For this review, take the finished solid that the model builds, in its own axes (mm). Face numbers are marked on the shaded views. A direction names the side the tool comes from. Coordinates: 2 decimals unless noted, no trailing zeros. Write each loop counter-clockwise with the first axis right and the second up, starting at its lowest first coordinate (ties: lowest second). Pieces come first, ordered by that corner, then holes. Notation, with made-up numbers: (6.25, -12.75) -> (12.25, -12.75) arc R23 cw to (12.25, 4.25) -> close; hole circle Ø2 at (11.25, 50). An arc over 180 degrees is marked (long way). Put each result on its own line as item: value. Start each with the question number.
Item 1: Insertion check: P1, Ø3, axis at x = 47.5, y = 2, coming from the -Z side; P2, Ø1, axis at y = 2.5, z = -10.5, coming from the +X side; P3, Ø3, axis at y = -2.5, z = 2.5, coming from the -X side. Each pin has a flat end and moves straight along its axis. Give the tip position at first contact, or say it passes through.
Item 2: Consider section B-B on y = -1. Give the boundary of the cut face in (x, z), and give its area (3 significant figures).
Item 3: Consider section C-C on x = 14. Give the boundary of the cut face in (y, z) (3 decimals).
Item 4: The part is to be moulded in two halves that separate along X. For the marked faces 3, 4 and 5, say which applies: +X half, -X half, draft (parallel to the pull), parting line (faces both ways), or undercut.
Item 5: To check wall thickness, follow L1, parallel to Z at x = 33.5, y = 1.5; L2, parallel to Z at x = 3, y = -0.5. State the ranges of each line that lie inside material, in increasing order.
Item 6: Consider section A-A on z = 0. Give the boundary of the cut face in (x, y) (3 decimals), and give its area (3 significant figures).
Item 7: Consider section D-D on x = 67.5. Give the boundary of the cut face in (y, z) (3 decimals).
Item 8: For the marked faces 1 and 2, list the 3-axis set-ups (+Z, -Z, +X, -X, +Y, -Y) from which the entire face can be reached by the end or side of a thin tool; tool diameter is ignored.
```python
from build123d import *

# Parameters (mm, degrees)
SKETCH1_R           = 3.2639
BOSS_EXTRUDE1_DEPTH = 3.175
BOSS_EXTRUDE2_START = -6.35
SKETCH3_R           = 2.4892
BOSS_EXTRUDE2_DEPTH = 6.35
FILLET2_R           = 6.35


with BuildPart() as part:
    # Sketch1 → Boss-Extrude1 (new, symmetric)
    with BuildSketch(Plane(origin=(0, 0, 0), x_dir=(1, 0, 0), z_dir=(0, 1, 0))):
        with BuildLine():
            Line((0, 6.35), (50.8, 6.35))
            ThreePointArc((50.8, 6.35), (57.15, 0), (50.8, -6.35))
            Line((50.8, -6.35), (0, -6.35))
            ThreePointArc((0, -6.35), (-6.35, 0), (0, 6.35))
        make_face()
        with Locations(Location((0, 0, 0), (0, 0, 270))):
            Circle(SKETCH1_R, mode=Mode.SUBTRACT)
        with Locations(Location((50.8, 0, 0), (0, 0, 270))):
            Circle(SKETCH1_R, mode=Mode.SUBTRACT)
    extrude(amount=BOSS_EXTRUDE1_DEPTH, both=True)

    # Sketch3 → Boss-Extrude2 (add)
    with BuildSketch(Plane.XZ.offset(3.175).offset(BOSS_EXTRUDE2_START)):
        with BuildLine():
            Line((76.840020478, -2.720263498), (52.97182791, 5.967048142))
            ThreePointArc((52.97182791, 5.967048142), (57.053529232, -1.102665928), (50.8, -6.35))
            Line((50.8, -6.35), (49.680323673, -6.35))
            Line((49.680323673, -6.35), (72.496364658, -14.654359782))
            ThreePointArc((72.496364658, -14.654359782), (80.63524071, -10.859139551), (76.840020478, -2.720263498))
        make_face()
        with Locations(Location((74.668192568, -8.68731164, 0), (0, 0, 270))):
            Circle(SKETCH3_R, mode=Mode.SUBTRACT)
    extrude(amount=BOSS_EXTRUDE2_DEPTH)

    # Fillet2
    fillet2_edges = [part.edges().sort_by_distance(p)[0] for p in [
        (49.680323673, 0, -6.35),
    ]]
    fillet(fillet2_edges, radius=FILLET2_R)


solid = part.part
```
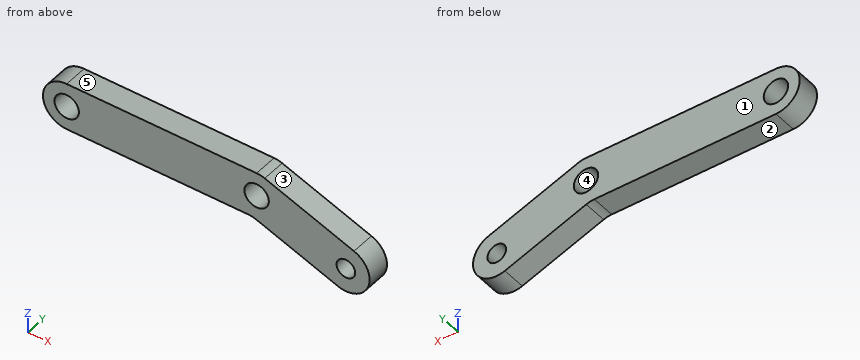
Return value:
1. P1: z = -6.37
1. P2: x = 80.88
1. P3: x = -6.27
2. outline: (0, -6.35) -> (48.56, -6.35) arc R6.35 cw to (50.73, -6.73) -> (72.5, -14.65) arc R6.35 ccw to (76.84, -2.72) -> (52.97, 5.97) arc R6.35 ccw to (50.8, 6.35) -> (0, 6.35) arc R6.35 ccw to start; hole circle Ø6.53 at (0, 0); hole circle Ø6.53 at (50.8, 0); hole circle Ø4.98 at (74.67, -8.69)
2. area: 1,010 mm^2
3. outline: (-3.175, -6.35) -> (3.175, -6.35) -> (3.175, 6.35) -> (-3.175, 6.35) -> close
4. face 3: +X half
4. face 4: undercut
4. face 5: draft
5. L1: -6.35 to 6.35
5. L2: -6.35 to -1.29, 1.29 to 6.35
6. outline: (-6.35, -3.175) -> (-3.264, -3.175) -> (-3.264, 3.175) -> (-6.35, 3.175) -> close; (3.264, -3.175) -> (47.536, -3.175) -> (47.536, 3.175) -> (3.264, 3.175) -> close; (54.064, -3.175) -> (69.366, -3.175) -> (69.366, 3.175) -> (54.064, 3.175) -> close
6. area: 398 mm^2
7. outline: (-3.175, -12.836) -> (3.175, -12.836) -> (3.175, 0.679) -> (-3.175, 0.679) -> close
8. face 1: +Z, -Z, +X, -X, +Y
8. face 2: -Z, -X, +Y, -Y
